Autodesk Inventor part; units mm, degrees
sketch "Sketch14" plane through (0, 0, 0) normal (0, 0, 1) x (1, 0, 0)
  line L0 (12, -11.25) -> (12, 11.25)
  line L1 (-12, 11.25) -> (-12, -11.25)
  line L2 (-12, -11.25) -> (12, 11.25) construction
  line L3 (12, -11.25) -> (-12, 11.25) construction
  line L4 (-12, 11.25) -> (5, 11.25)
  line L5 (5, 11.25) -> (5, 16.25)
  line L6 (5, 16.25) -> (7.3, 16.25)
  line L7 (7.3, 16.25) -> (7.3, 11.25)
  line L8 (5, -11.25) -> (5, -16.25)
  line L9 (5, -16.25) -> (7.3, -16.25)
  line L10 (7.3, -16.25) -> (7.3, -11.25)
  line L11 (7.3, 11.25) -> (12, 11.25)
  line L12 (7.3, -11.25) -> (12, -11.25)
  line L13 (-12, -11.25) -> (5, -11.25)
  line L14 (7.3, -11.25) -> (7.3, -16.25)
  line L15 (5, -16.25) -> (5, -11.25)
  line L16 (-12, -11.25) -> (-12, 11.25)
  line L17 (5, 11.25) -> (-12, 11.25)
  line L18 (-12, -11.25) -> (5, -11.25)
  line L19 (5, -11.25) -> (5, -16.25)
  line L20 (7.3, -11.25) -> (12, -11.25)
  line L21 (12, 11.25) -> (7.3, 11.25)
  line L22 (-12, 11.25) -> (12, 11.25)
  line L23 (12, 11.25) -> (12, -11.25)
  line L24 (12, -11.25) -> (-12, -11.25)
  line L25 (-12, -11.25) -> (-12, 11.25)
  line L26 (5, 16.25) -> (7.3, 16.25)
  line L27 (7.3, 16.25) -> (7.3, 11.25)
  line L28 (7.3, 11.25) -> (5, 11.25)
  line L29 (5, 11.25) -> (5, 16.25)
  line L30 (5, -11.25) -> (7.3, -11.25)
  line L31 (7.3, -11.25) -> (7.3, -16.25)
  line L32 (7.3, -16.25) -> (5, -16.25)
  line L33 (5, -16.25) -> (5, -11.25)
  point P0 (0, 0)
  dimension "d105" = 24
  dimension "d106" = 22.5
  dimension "d107" = 17
  dimension "d108" = 5
  dimension "d109" = 2.3
extrude "Extrusion12" add sketch "Sketch14" along normal blind 12
sketch "Sketch15" plane through (12, -11.25, 0) normal (1, 0, 0) x (0, 0, -1)
  line L0 (0, 0) -> (0, -5)
  line L1 (0, -5) -> (-6, -5)
  line L2 (0, -5) -> (-12, -5)
  line L3 (-6, -5) -> (-6, 5.75)
  circle A0 centre (-6, 5.75) radius 5.75
  point P0 (0, 11.25)
  dimension "d112" = 10.75
  dimension "d113" = 11.5
extrude "Extrusion13" add sketch "Sketch15" along normal blind 4
sketch "Sketch16" plane through (16, -5.5, 6) normal (1, 0, 0) x (0, 0, -1)
  circle A0 centre (0, 0) radius 5.75
  circle A1 centre (0, 0) radius 2.5
  point P0 (6, 5.5)
  dimension "d116" = 5
extrude "Extrusion14" add sketch "Sketch16" along normal blind 3 contours A1
sketch "Sketch18" plane through (0, 0, 12) normal (0, 0, 1) x (1, 0, 0)
  line L0 (-10.7887, 4.9339) -> (3.2892, 4.9339) construction
  line L1 (3.2892, 4.9339) -> (3.2892, -9.473) construction
  line L2 (3.2892, -9.473) -> (-10.7887, -9.473) construction
  line L3 (-10.7887, -9.473) -> (-10.7887, 4.9339) construction
  point P0 (0, 0)
properties part number "Motor Waterkanon" material "S235"
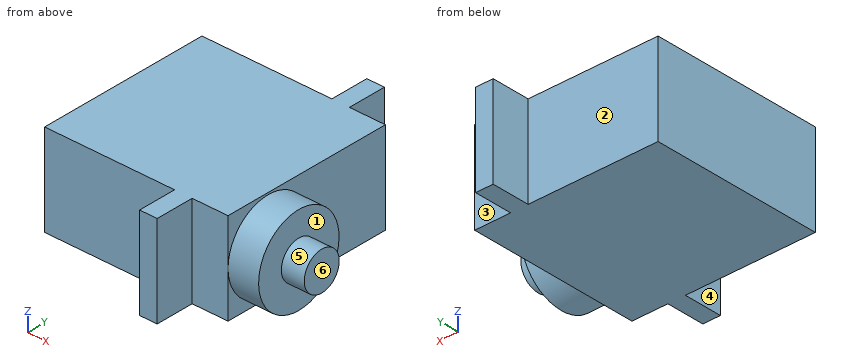
The model under review builds one solid part; all positions refer to its coordinate system, in mm. Face numbers are marked on the shaded views. A direction names the side the tool comes from. Round coordinates to 2 decimals unless told otherwise and drop trailing zeros. Loops run counter-clockwise (first coordinate to the right, second up) from the corner with the lowest first, then second, coordinate; pieces in that order, holes last.
Item 1: For the marked faces 1, 2 and 3, list the 3-axis set-ups (+Z, -Z, +X, -X, +Y, -Y) from which the entire face can be reached by the end or side of a thin tool; tool diameter is ignored.
Determined:
face 1: +X
face 2: +Z, -Z, -X, +Y
face 3: +Z, -Z, +X, +Y
Item 2: Take a section at D-D (z = 1.25). Write out the cut boundary in (x, y).
Determined:
outline: (-12, -11.25) - (5, -11.25) - (5, -16.25) - (7.3, -16.25) - (7.3, -11.25) - (12, -11.25) - (12, -8.74) - (16, -8.74) - (16, -2.26) - (12, -2.26) - (12, 11.25) - (7.3, 11.25) - (7.3, 16.25) - (5, 16.25) - (5, 11.25) - (-12, 11.25) - close
Item 3: Take a section at A-A (y = -5.5). Write out the cut boundary in (x, z), then the cut area to 3 significant figures.
Determined:
outline: (-12, 0) - (12, 0) - (12, 0.25) - (16, 0.25) - (16, 3.5) - (19, 3.5) - (19, 8.5) - (16, 8.5) - (16, 11.75) - (12, 11.75) - (12, 12) - (-12, 12) - close
area: 349 mm2
Item 4: Mouldability with a two-part tool opening along X and no side actions: class the marked faces 4, 5 and 6 as released by +X, released by -X, zero draft, split by the parting line, or undercut.
Determined:
face 4: released by -X
face 5: zero draft
face 6: released by +X
Item 5: Take a section at B-B (z = 4.25). Write out the cut boundary in (x, y), then the cut area to 3 significant figures.
Determined:
outline: (-12, -11.25) - (5, -11.25) - (5, -16.25) - (7.3, -16.25) - (7.3, -11.25) - (12, -11.25) - (12, -10.98) - (16, -10.98) - (16, -7.29) - (19, -7.29) - (19, -3.71) - (16, -3.71) - (16, -0.02) - (12, -0.02) - (12, 11.25) - (7.3, 11.25) - (7.3, 16.25) - (5, 16.25) - (5, 11.25) - (-12, 11.25) - close
area: 618 mm2
Item 6: Take a section at C-C (x = 15). Write out the cut boundary in (y, z).
Determined:
outline: circle Ø11.5 at (-5.5, 6)
Item 7: Clearance check with flat-ended pins moving along their axes: pin 1 Ø3.5 at (x, z) = (-5, 5.5) entering from -Y; pin 2 Ø3 at (x, z) = (-0.5, 10) entering from +Y; pin 3 Ø5.5 at (y, z) = (14.5, 8.5) entering from -X. State where each tip first meets the part, or that it passes through.
Determined:
pin 1: stops at y = -11.25
pin 2: stops at y = 11.25
pin 3: stops at x = 5
Item 8: For line 1 (X direction, y = 9, z = 4); line 2 (X direction, y = -12, z = 2.25); line 3 (Y direction, x = -3, z = 1.25), list the stretches that pass through material, from the lowest coordinate up.
Determined:
line 1: x = -12 to 12
line 2: x = 5 to 7.3
line 3: y = -11.25 to 11.25
